from build123d import *

# Parameters (mm, degrees)
AUFSATZ_LINEAR_AUSTRAGEN1_DEPTH = 6
AUFSATZ_LINEAR_AUSTRAGEN2_DEPTH = 2
SKIZZE3_OUTSIDE_W               = 126.466
SKIZZE3_OUTSIDE_H               = 96.466
SKIZZE3_OUTSIDE_W_2             = 100
SKIZZE3_OUTSIDE_H_2             = 70
SKIZZE3_OUTSIDE_R               = 2.1
SCHNITT_LINEAR_AUSTRAGEN1_DEPTH = 6
SKIZZE4_R                       = 4.2
SCHNITT_LINEAR_AUSTRAGEN2_DEPTH = 4
SKIZZE5_R                       = 3.95
SKIZZE5_R_2                     = 1.45
AUFSATZ_LINEAR_AUSTRAGEN3_DEPTH = 20


with BuildPart() as part:
    # Skizze1 → Aufsatz-Linear austragen1 (new body)
    with BuildSketch(Plane(origin=(0, 0, 0), x_dir=(1, 0, 0), z_dir=(0, 1, 0))):
        Polygon((-50, -35), (50, -35), (50, 35), (-15.02457838, 35), (-35.02457838, 35), (-50, 35), align=None)
    extrude(amount=AUFSATZ_LINEAR_AUSTRAGEN1_DEPTH)

    # Skizze2 → Aufsatz-Linear austragen2 (add)
    with BuildSketch(Plane(origin=(0, 0, 0), x_dir=(-1, 0, 0), z_dir=(0, -1, 0))):
        with BuildLine():
            Line((39.65, -32.75), (-39.65, -32.75))
            Line((-39.65, -32.75), (-39.65, -30))
            ThreePointArc((-39.65, -30), (-41.216978721, -26.216978721), (-45, -24.65))
            Line((-45, -24.65), (-47.75, -24.65))
            Line((-47.75, -24.65), (-47.75, 24.65))
            Line((-47.75, 24.65), (-45, 24.65))
            ThreePointArc((-45, 24.65), (-41.216978721, 26.216978721), (-39.65, 30))
            Line((-39.65, 30), (-39.65, 32.75))
            Line((-39.65, 32.75), (39.65, 32.75))
            Line((39.65, 32.75), (39.65, 30))
            ThreePointArc((39.65, 30), (41.216978721, 26.216978721), (45, 24.65))
            Line((45, 24.65), (47.75, 24.65))
            Line((47.75, 24.65), (47.75, -24.65))
            Line((47.75, -24.65), (45, -24.65))
            ThreePointArc((45, -24.65), (41.216978721, -26.216978721), (39.65, -30))
            Line((39.65, -30), (39.65, -32.75))
        make_face()
        with BuildLine():
            Line((45.75, 22.65), (45.75, -22.65))
            Line((45.75, -22.65), (45, -22.65))
            ThreePointArc((45, -22.65), (39.802765158, -24.802765158), (37.65, -30))
            Line((37.65, -30), (37.65, -30.75))
            Line((37.65, -30.75), (-37.65, -30.75))
            Line((-37.65, -30.75), (-37.65, -30))
            ThreePointArc((-37.65, -30), (-39.802765158, -24.802765158), (-45, -22.65))
            Line((-45, -22.65), (-45.75, -22.65))
            Line((-45.75, -22.65), (-45.75, 22.65))
            Line((-45.75, 22.65), (-45, 22.65))
            ThreePointArc((-45, 22.65), (-39.802765158, 24.802765158), (-37.65, 30))
            Line((-37.65, 30), (-37.65, 30.75))
            Line((-37.65, 30.75), (37.65, 30.75))
            Line((37.65, 30.75), (37.65, 30))
            ThreePointArc((37.65, 30), (39.802765158, 24.802765158), (45, 22.65))
            Line((45, 22.65), (45.75, 22.65))
        make_face(mode=Mode.SUBTRACT)
    extrude(amount=AUFSATZ_LINEAR_AUSTRAGEN2_DEPTH)

    # Skizze3 outside → Schnitt-Linear austragen1 (cut)
    # profile 1 of 5: a face of its own
    with BuildSketch(Plane(origin=(0, 6, 0), x_dir=(1, 0, 0), z_dir=(0, 1, 0))):
        Rectangle(SKIZZE3_OUTSIDE_W, SKIZZE3_OUTSIDE_H)
        Rectangle(SKIZZE3_OUTSIDE_W_2, SKIZZE3_OUTSIDE_H_2, mode=Mode.SUBTRACT)
    # profile 2 of 5: a face of its own
    with BuildSketch(Plane(origin=(0, 6, 0), x_dir=(1, 0, 0), z_dir=(0, 1, 0))):
        with Locations(Location((-45, -30, 0), (0, 0, 270))):
            Circle(SKIZZE3_OUTSIDE_R)
    # profile 3 of 5: a face of its own
    with BuildSketch(Plane(origin=(0, 6, 0), x_dir=(1, 0, 0), z_dir=(0, 1, 0))):
        with Locations(Location((-45, 30, 0), (0, 0, 270))):
            Circle(SKIZZE3_OUTSIDE_R)
    # profile 4 of 5: a face of its own
    with BuildSketch(Plane(origin=(0, 6, 0), x_dir=(1, 0, 0), z_dir=(0, 1, 0))):
        with Locations(Location((45, -30, 0), (0, 0, 270))):
            Circle(SKIZZE3_OUTSIDE_R)
    # profile 5 of 5: a face of its own
    with BuildSketch(Plane(origin=(0, 6, 0), x_dir=(1, 0, 0), z_dir=(0, 1, 0))):
        with Locations(Location((45, 30, 0), (0, 0, 270))):
            Circle(SKIZZE3_OUTSIDE_R)
    extrude(amount=-SCHNITT_LINEAR_AUSTRAGEN1_DEPTH, mode=Mode.SUBTRACT)

    # Skizze4 → Schnitt-Linear austragen2 (cut)
    with BuildSketch(Plane(origin=(0, 6, 0), x_dir=(1, 0, 0), z_dir=(0, 1, 0))):
        with Locations(Location((-45, -30, 0), (0, 0, 270))):
            Circle(SKIZZE4_R)
        with Locations(Location((45, -30, 0), (0, 0, 270))):
            Circle(SKIZZE4_R)
        with Locations(Location((45, 30, 0), (0, 0, 270))):
            Circle(SKIZZE4_R)
        with Locations(Location((-45, 30, 0), (0, 0, 270))):
            Circle(SKIZZE4_R)
    extrude(amount=-SCHNITT_LINEAR_AUSTRAGEN2_DEPTH, mode=Mode.SUBTRACT)

    # Skizze5 → Aufsatz-Linear austragen3 (add)
    # profile 1 of 4: a face of its own
    with BuildSketch(Plane(origin=(0, 0, 0), x_dir=(-1, 0, 0), z_dir=(0, -1, 0))):
        with Locations(Location((25, -20, 0), (0, 0, 270))):
            Circle(SKIZZE5_R)
        with Locations(Location((25, -20, 0), (0, 0, 90))):
            Circle(SKIZZE5_R_2, mode=Mode.SUBTRACT)
    # profile 2 of 4: a face of its own
    with BuildSketch(Plane(origin=(0, 0, 0), x_dir=(-1, 0, 0), z_dir=(0, -1, 0))):
        with Locations(Location((-25, -20, 0), (0, 0, 270))):
            Circle(SKIZZE5_R)
        with Locations(Location((-25, -20, 0), (0, 0, 270))):
            Circle(SKIZZE5_R_2, mode=Mode.SUBTRACT)
    # profile 3 of 4: a face of its own
    with BuildSketch(Plane(origin=(0, 0, 0), x_dir=(-1, 0, 0), z_dir=(0, -1, 0))):
        with Locations(Location((-25, 20, 0), (0, 0, 270))):
            Circle(SKIZZE5_R)
        with Locations(Location((-25, 20, 0), (0, 0, 90))):
            Circle(SKIZZE5_R_2, mode=Mode.SUBTRACT)
    # profile 4 of 4: a face of its own
    with BuildSketch(Plane(origin=(0, 0, 0), x_dir=(-1, 0, 0), z_dir=(0, -1, 0))):
        with Locations(Location((25, 20, 0), (0, 0, 270))):
            Circle(SKIZZE5_R)
        with Locations(Location((25, 20, 0), (0, 0, 270))):
            Circle(SKIZZE5_R_2, mode=Mode.SUBTRACT)
    extrude(amount=AUFSATZ_LINEAR_AUSTRAGEN3_DEPTH)


solid = part.part
Source: CAD feature listing. Evaluate the final solid. Frame: model axes, mm. A direction names the side the tool comes from. Give positions to 0.01 mm unless a question says otherwise; leave off trailing zeros. Order: outer loops, then holes, each group sorted by start corner. A loop starts at its lowest first (then second) coordinate and runs counter-clockwise, first axis right, second up. Notation, with made-up numbers: (-22.5, 49.25) -> (-4.5, 49.25) arc R17 ccw to (-4.5, 76.25) -> close; hole circle Ø7 at (87, -19). An arc over 180 degrees is marked (long way). Write item = value, one per line.
Item 1: Contact query for flat-ended pins moving along their axis: pin 1 (4 mm diameter, centred on y = -12.5, z = 26, fed in from -X); pin 2 (0.6 mm diameter, centred on y = -1, z = 31.5, fed in from +X); pin 3 (12 mm diameter, centred on x = -15.5, y = -6.5, fed in from -Z); pin 4 (8 mm diameter, centred on x = -30.5, y = -9, fed in from -Z). Output: stop coordinate, or through.
Check result:
pin_1 = through
pin_2 = 39.65
pin_3 = -32.75
pin_4 = -23.65
Item 2: Ray query, probe 1 along X at (y, z) = (-8.5, -20); probe 2 along X at (y, z) = (0.75, -30); probe 3 along X at (y, z) = (2.9, -30). Return the intervals inside material, ascending.
Check result:
probe_1 = -28.95 to -26.45, -23.55 to -21.05, 21.05 to 23.55, 26.45 to 28.95
probe_2 = -50 to -47.1, -42.9 to 42.9, 47.1 to 50
probe_3 = -50 to -49.2, -40.8 to 40.8, 49.2 to 50
Item 3: Set-up query: faces 1 (the face through (46, -1, -24.65)), 2 (the face through (-47, 2, 32)), 3 (the face through (41.176, -0.986, 26.259)), 4 (the face through (-25, 0, -20)), 5 (the face through (25, -20, 22)). Return all of +Z, -Z, +X, -X, +Y, -Y with unobstructed straight access to the full face (end or side cutting, diameter ignored); none if empty.
Check result:
face_1 = -Z, +X, -Y
face_2 = +Y
face_3 = +Z, +X, -Y
face_4 = -Y
face_5 = +Z, -Z, +X, -X, -Y
Item 4: Section query B-B (x = 33.5). Output: boundary loops of the cut face in (y, z).
Check result:
outline = (-2, -32.75) -> (0, -32.75) -> (0, -35) -> (6, -35) -> (6, 35) -> (0, 35) -> (0, 32.75) -> (-2, 32.75) -> (-2, 30.75) -> (0, 30.75) -> (0, -30.75) -> (-2, -30.75) -> close
Item 5: Section query D-D (x = -25). Output: boundary loops of the cut face in (y, z).
Check result:
outline = (-20, -23.95) -> (0, -23.95) -> (0, -30.75) -> (-2, -30.75) -> (-2, -32.75) -> (0, -32.75) -> (0, -35) -> (6, -35) -> (6, 35) -> (0, 35) -> (0, 32.75) -> (-2, 32.75) -> (-2, 30.75) -> (0, 30.75) -> (0, 23.95) -> (-20, 23.95) -> (-20, 21.45) -> (0, 21.45) -> (0, 18.55) -> (-20, 18.55) -> (-20, 16.05) -> (0, 16.05) -> (0, -16.05) -> (-20, -16.05) -> (-20, -18.55) -> (0, -18.55) -> (0, -21.45) -> (-20, -21.45) -> close
Item 6: Mould query, pull axis X, two halves, no side actions, for faces 6 (the face through (25.555, -9.86, 21.339)), 7 (the face through (46, -1, 24.65)), 8 (the face through (-45.75, -1, 0)), 9 (the face through (-47.75, -1, 0)). Classes: +X half, -X half, draft (parallel to the pull), parting line (faces both ways), or undercut.
Check result:
face_6 = undercut
face_7 = draft
face_8 = undercut
face_9 = -X half
Item 7: Section query A-A (y = -15.5). Output: boundary loops of the cut face in (x, z).
Check result:
outline = circle Ø7.9 at (-25, -20); circle Ø7.9 at (-25, 20); circle Ø7.9 at (25, -20); circle Ø7.9 at (25, 20); hole circle Ø2.9 at (-25, -20); hole circle Ø2.9 at (-25, 20); hole circle Ø2.9 at (25, -20); hole circle Ø2.9 at (25, 20)
Item 8: Section query C-C (z = 20). Output: boundary loops of the cut face in (x, y).
Check result:
outline = (-50, 0) -> (-47.75, 0) -> (-47.75, -2) -> (-45.75, -2) -> (-45.75, 0) -> (-28.95, 0) -> (-28.95, -20) -> (-26.45, -20) -> (-26.45, 0) -> (-23.55, 0) -> (-23.55, -20) -> (-21.05, -20) -> (-21.05, 0) -> (21.05, 0) -> (21.05, -20) -> (23.55, -20) -> (23.55, 0) -> (26.45, 0) -> (26.45, -20) -> (28.95, -20) -> (28.95, 0) -> (45.75, 0) -> (45.75, -2) -> (47.75, -2) -> (47.75, 0) -> (50, 0) -> (50, 6) -> (-50, 6) -> close
